Geometry check sheet. Reference: the model listing, model coordinates, mm. Face numbers are marked on the shaded views. A direction names the side the tool comes from. Round coordinates to 2 decimals unless told otherwise and drop trailing zeros. Order: outer loops, then holes, each group sorted by start corner. A loop starts at its lowest first (then second) coordinate and runs counter-clockwise, first axis right, second up.
(1) Gauge pin test, flat ends, axial feed: P1, Ø3, axis at y = 13.5, z = -4.5, coming from the +X side; P2, Ø3.5, axis at x = 52.455, z = 3.955, coming from the -Y side; P3, Ø5, axis at y = 11.5, z = 6, coming from the -X side. Record the tip position at first contact, or that the pin passes through.
(2) Set-up check for the marked faces 1 and 2: record each of +Z, -Z, +X, -X, +Y, -Y from which the full face is reachable in a straight line by a thin tool's end or side.
(3) Cross-section at C-C on z = 9.75. Enter the section's corners in (x, y), and give its area (3 significant figures).
(4) Cross-section at A-A on z = -5. Enter the section's corners in (x, y).
(5) Cross-section at B-B on y = 2.25. Enter the section's corners in (x, z) (3 decimals), and give its area (3 significant figures).
(6) Cross-section at D-D on x = 49. Enter the section's corners in (y, z), and give its area (3 significant figures).
(7) Thickness scan on L1, parallel to X at y = 2, z = -4.25; L2, parallel to X at y = 4.25, z = 5; L3, parallel to Y at x = -50, z = 9.75. Record the ranges inside material, lowest first.
from build123d import *

# Parameters (mm, degrees)
SKETCH1_W           = 112.1
SKETCH1_H           = 22
SKETCH1_R           = 2.025
BOSS_EXTRUDE1_DEPTH = 6.5
SKETCH2_W           = 94.239862036
SKETCH2_H           = 22
BOSS_EXTRUDE3_DEPTH = 9.5


with BuildPart() as part:
    # Sketch1 → Boss-Extrude1 (new body)
    with BuildSketch(Plane(origin=(0, 0, 0), x_dir=(1, 0, 0), z_dir=(0, 1, 0))):
        Rectangle(SKETCH1_W, SKETCH1_H)
        with Locations((-52.455, 3.955)):
            Circle(SKETCH1_R, mode=Mode.SUBTRACT)
        with Locations((-52.455, -3.955)):
            Circle(SKETCH1_R, mode=Mode.SUBTRACT)
        with Locations((52.455, -3.955)):
            Circle(SKETCH1_R, mode=Mode.SUBTRACT)
        with Locations((52.455, 3.955)):
            Circle(SKETCH1_R, mode=Mode.SUBTRACT)
    extrude(amount=BOSS_EXTRUDE1_DEPTH)

    # Sketch2 → Boss-Extrude3 (add)
    with BuildSketch(Plane(origin=(0, 6.5, 0), x_dir=(1, 0, 0), z_dir=(0, 1, 0))):
        Rectangle(SKETCH2_W, SKETCH2_H)
    extrude(amount=BOSS_EXTRUDE3_DEPTH)


solid = part.part
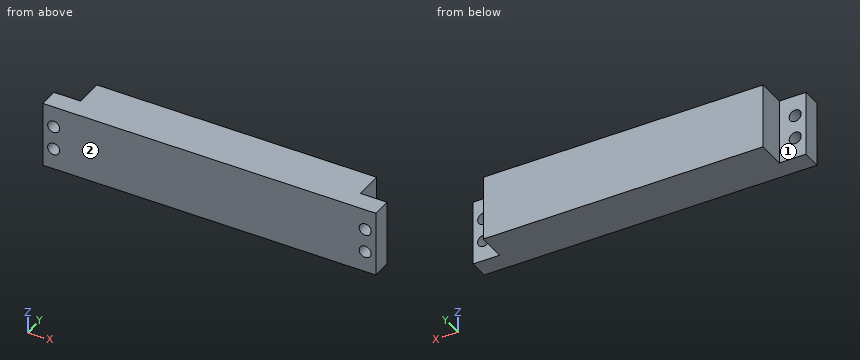
Found:
1. P1: stops at x = 47.12
1. P2: passes through
1. P3: stops at x = -47.12
2. face 1: +Z, -Z, -X, +Y
2. face 2: +Z, -Z, +X, -X, -Y
3. outline: (-56.05, 0) - (56.05, 0) - (56.05, 6.5) - (47.12, 6.5) - (47.12, 16) - (-47.12, 16) - (-47.12, 6.5) - (-56.05, 6.5) - close
3. area: 1,620 mm2
4. outline: (-56.05, 0) - (-54.19, 0) - (-54.19, 6.5) - (-56.05, 6.5) - close; (-50.72, 0) - (50.72, 0) - (50.72, 6.5) - (47.12, 6.5) - (47.12, 16) - (-47.12, 16) - (-47.12, 6.5) - (-50.72, 6.5) - close; (54.19, 0) - (56.05, 0) - (56.05, 6.5) - (54.19, 6.5) - close
5. outline: (-56.05, -11) - (56.05, -11) - (56.05, 11) - (-56.05, 11) - close; hole circle Ø4.05 at (-52.455, -3.955); hole circle Ø4.05 at (-52.455, 3.955); hole circle Ø4.05 at (52.455, -3.955); hole circle Ø4.05 at (52.455, 3.955)
5. area: 2,410 mm2
6. outline: (0, -11) - (6.5, -11) - (6.5, 11) - (0, 11) - close
6. area: 143 mm2
7. L1: x = -56.05 to -54.46, -50.45 to 50.45, 54.46 to 56.05
7. L2: x = -56.05 to -54.19, -50.72 to 50.72, 54.19 to 56.05
7. L3: y = 0 to 6.5
